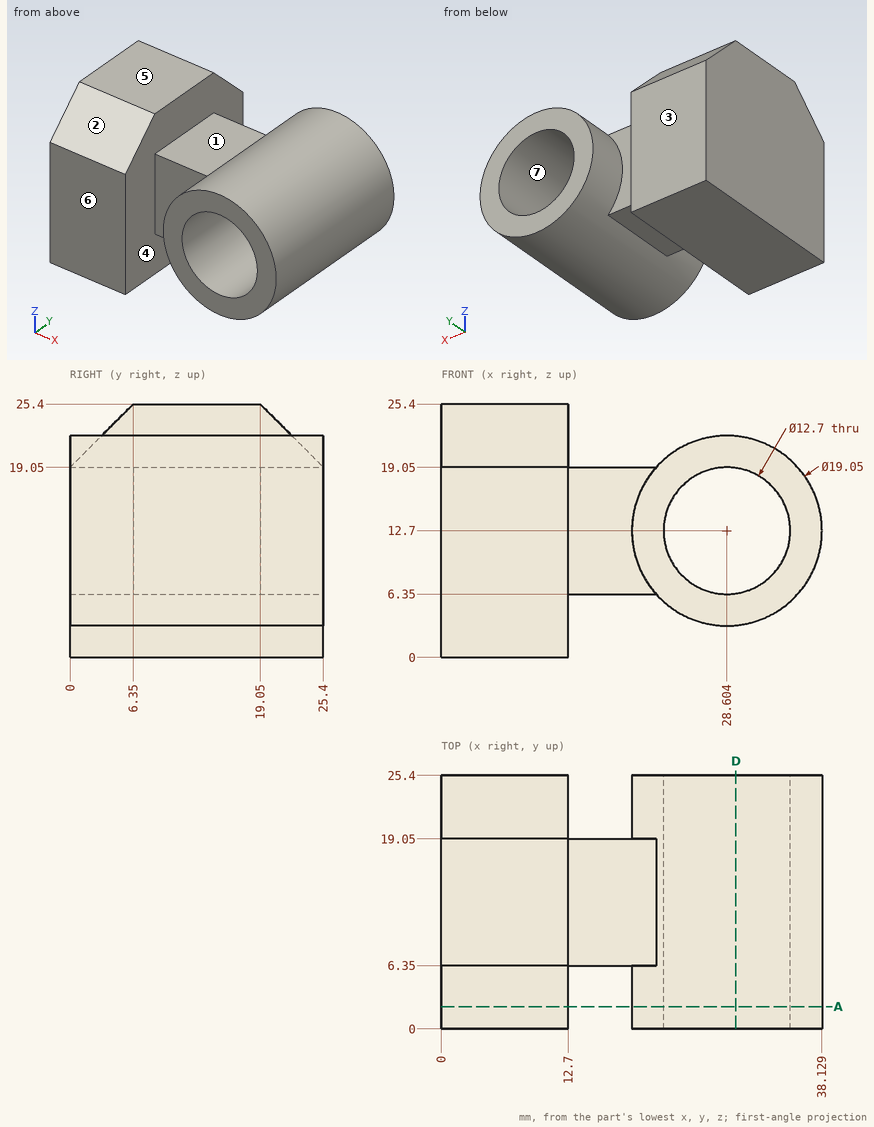
The drawing under review shows one solid part. Ordinate dimensions are in mm from its lowest x, y, z. A direction names the side the tool comes from. Coordinates: 2 decimals unless noted, no trailing zeros. Write each loop counter-clockwise with the first axis right and the second up, starting at its lowest first coordinate (ties: lowest second). Pieces come first, ordered by that corner, then holes. Notation, with made-up numbers: (42, 43) - (47, 43) arc R33 ccw to (47, 78) - close; hole circle Ø4 at (-12, 87). An arc over 180 degrees is marked (long way). Put each result on its own line as item: value.
1. Machinability: for the marked faces 1, 2, 3 and 4, which of the approach directions +Z, -Z, +X, -X, +Y, -Y give a long, thin tool a straight path to every point of the face, cutting with its end or side? Answer none if there is none.
Values found:
face 1: +Z, +Y, -Y
face 2: +Z, -X, -Y
face 3: +Z, -Z, +X, -X, +Y
face 4: none
2. Wall thickness on probe 1 along X at (y, z) = (4.25, 11) (1 decimal); probe 2 along X at (y, z) = (23.75, 12.25); probe 3 along Z at (x, y) = (24, 18) (1 decimal): over which ranges is each line inside the solid? List them lowest first.
Values found:
probe 1: 0 to 12.7, 19.2 to 22.5, 34.7 to 38
probe 2: 0 to 12.7, 19.09 to 22.27, 34.94 to 38.12
probe 3: 4.4 to 8.3, 17.1 to 21
3. For pin 1 (2.5 mm diameter, centred on x = 16, z = 10, fed in from +Y); pin 2 (1.5 mm diameter, centred on x = 32, y = 8, fed in from -Z); pin 3 (1 mm diameter, centred on x = 22, y = 17.5, fed in from +Z), all flat-tipped, find the tip position at first contact; note any pin that passes through.
Values found:
pin 1: y = 19.05
pin 2: z = 3.55
pin 3: z = 20.01
4. Add section D-D, the plane x = 29.5. Give the boundary of the cut face in (y, z).
Values found:
outline: (0, 3.22) - (25.4, 3.22) - (25.4, 6.41) - (0, 6.41) - close; (0, 18.99) - (25.4, 18.99) - (25.4, 22.18) - (0, 22.18) - close
5. Add section A-A, the plane y = 2.25. Count the separate pieces of the cut face and the enclosed holes in it, then the cut area to 3 significant figures.
Values found:
separate pieces: 2
enclosed holes: 1
area: 429 mm²
6. Mouldability with a two-part tool opening along Z and no side actions: class the marked faces 5, 6 and 7 as released by +Z, released by -Z, zero draft, split by the parting line, or undercut.
Values found:
face 5: released by +Z
face 6: zero draft
face 7: undercut
